```python
from build123d import *

# Parameters (mm, degrees)
SKETCH1_R            = 10
SKETCH1_R_2          = 9
BOSS_EXTRUDE1_DEPTH  = 166
M3_CLEARANCE_HOLE1_D = 3.6
CUT_EXTRUDE1_REACH   = 12
SKETCH7_R            = 1.5
SKETCH8_R            = 1.5
CUT_EXTRUDE2_DEPTH   = 11.0000001


with BuildPart() as part:
    # Sketch1 → Boss-Extrude1 (new body)
    with BuildSketch(Plane(origin=(0, 0, 0), x_dir=(1, 0, 0), z_dir=(0, 1, 0))):
        Circle(SKETCH1_R)
        Circle(SKETCH1_R_2, mode=Mode.SUBTRACT)
    extrude(amount=BOSS_EXTRUDE1_DEPTH)

    # M3 Clearance Hole1 (through all)
    with Locations(Plane(origin=(10, 0, 0), x_dir=(0, 0, -1), z_dir=(1, 0, 0))):
        with Locations((0, 5)):
            m3_clearance_hole1 = Hole(M3_CLEARANCE_HOLE1_D / 2)

    # Mirror1: M3 Clearance Hole1 across plane
    add(m3_clearance_hole1.mirror(Plane.ZX.offset(83)), mode=Mode.SUBTRACT)

    # Sketch7 → Cut-Extrude1 (cut, up to next)
    with BuildSketch(Plane.XY, mode=Mode.PRIVATE) as cut_extrude1_sk1:
        with Locations((0, 25)):
            Circle(SKETCH7_R)
    cut_extrude1_tool1 = extrude(cut_extrude1_sk1.sketch, amount=CUT_EXTRUDE1_REACH, mode=Mode.PRIVATE) & part.part
    add(cut_extrude1_tool1.solids().sort_by_distance((0, 25, 0))[0], mode=Mode.SUBTRACT)

    # Sketch8 → Cut-Extrude2 (cut, through all)
    with BuildSketch(Plane.XY):
        with Locations((0, 141)):
            Circle(SKETCH8_R)
    extrude(amount=-CUT_EXTRUDE2_DEPTH, mode=Mode.SUBTRACT)


solid = part.part
```
Check sheet for the modelled part. Datum: model origin and axes. Units: mm. A direction names the side the tool comes from. Round coordinates to 2 decimals unless told otherwise and drop trailing zeros. Order: outer loops, then holes, each group sorted by start corner. A loop starts at its lowest first (then second) coordinate and runs counter-clockwise, first axis right, second up.
1) Scan lines: line 1 (X direction, y = 45, z = 0); line 2 (Y direction, x = 0, z = 9.7); line 3 (Z direction, x = -0.5, y = 61). Record each from-to range of solid material in increasing order.
2) Section check A-A (z = 0). Record the boundary of the cut face in (x, y), and give its area (3 significant figures).
3) Section check C-C (y = 32). Record the boundary of the cut face in (x, z).
4) Mould release check, pull along Y, two halves, no side actions. Record for faces 4 (the cylindrical face through (9.401, 161.689, 1.663)), 5 (the flat face through (-9, 0, -2)), 6 (the flat face through (-9, 166, -2)): +Y half, -Y half, draft (parallel to the pull), parting line (faces both ways), or undercut.
5) Section check B-B (z = -6.25). Record the boundary of the cut face in (x, y), and give its area (3 significant figures).
6) Section check D-D (x = -5.75). Record the boundary of the cut face in (y, z), and give its area (3 significant figures).
7) Tool access check on faces 1 (the cylindrical face through (-0.195, 26.487, 9.429)), 2 (the cylindrical face through (-0.195, 142.487, -9.429)), 3 (the cylindrical face through (9.401, 5.541, 1.717)). Record the directions out of +Z, -Z, +X, -X, +Y, -Y that give a thin tool (end or side, any length) a straight path to the whole face; none if there is none.
8) Go/stop test with flat-tipped pins: pin 1 Ø3 at (y, z) = (5, 0) entering from +X; pin 2 Ø6 at (y, z) = (117.5, -7) entering from -X; pin 3 Ø6 at (y, z) = (143, -5) entering from -X; pin 4 Ø6 at (y, z) = (125, 3.5) entering from +X. Record where each tip stops, or that it passes through.
Result:
1. line 1: x = -10 to -9, 9 to 10
1. line 2: y = 0 to 23.5, 26.5 to 166
1. line 3: z = -9.99 to -8.99, 8.99 to 9.99
2. outline: (-10, 0) - (-9, 0) - (-9, 3.2) - (-10, 3.2) - close; (-10, 6.8) - (-9, 6.8) - (-9, 159.2) - (-10, 159.2) - close; (-10, 162.8) - (-9, 162.8) - (-9, 166) - (-10, 166) - close; (9, 0) - (10, 0) - (10, 3.2) - (9, 3.2) - close; (9, 6.8) - (10, 6.8) - (10, 159.2) - (9, 159.2) - close; (9, 162.8) - (10, 162.8) - (10, 166) - (9, 166) - close
2. area: 318 mm2
3. outline: circle Ø20 at (0, 0); hole circle Ø18 at (0, 0)
4. face 4: undercut
4. face 5: -Y half
4. face 6: +Y half
5. outline: (-7.81, 0) - (-6.48, 0) - (-6.48, 166) - (-7.81, 166) - close; (6.48, 0) - (7.81, 0) - (7.81, 166) - (6.48, 166) - close
5. area: 442 mm2
6. outline: (0, -8.18) - (166, -8.18) - (166, -6.92) - (0, -6.92) - close; (0, 6.92) - (166, 6.92) - (166, 8.18) - (0, 8.18) - close
6. area: 418 mm2
7. face 1: +Z
7. face 2: -Z
7. face 3: +X, -X
8. pin 1: passes through
8. pin 2: stops at x = -9.17
8. pin 3: stops at x = -9.8
8. pin 4: stops at x = 9.99
